Geometry check sheet. Reference: drawing and pictorial views, mm from the part's lowest x, y, z. Round coordinates to 2 decimals unless told otherwise and drop trailing zeros. Write each loop counter-clockwise with the first axis right and the second up, starting at its lowest first coordinate (ties: lowest second). Pieces come first, ordered by that corner, then holes.
Item 1: Section check A-A, the plane z = 17. Record the cut outline in (x, y).
Item 2: Section check B-B, the plane x = 17. Record the cut outline in (y, z).
Item 3: Section check D-D, the plane y = 4.75. Record the cut outline in (x, z), plus the area to 3 significant figures.
Item 4: Section check C-C, the plane y = 0.75. Record the cut outline in (x, z), plus the area to 3 significant figures.
Item 5: Material ranges on line 1 along Z through (x, y) = (17, 2.45); line 2 along Z through (x, y) = (17, 5.3), recorded low to high.
Item 6: Release check for a two-part mould opening along Z. For the marked faces 1, 2 and 3 record: pulls with the +Z half, pulls with the -Z half, needs draft (parallel to the pull), parting line crosses it, or undercut.
Item 7: Depth check by flat-ended pin: pin 1 (10 mm diameter, centred on x = 10, z = 18.5, fed in from +Y); pin 2 (2 mm diameter, centred on x = 30, z = 18.5, fed in from -Y); pin 3 (2 mm diameter, centred on y = 5, z = 9.5, fed in from -X); pin 4 (1.5 mm diameter, centred on y = 5.5, z = 14, fed in from +X). Enter the tip coordinate at first touch or a pass-through.
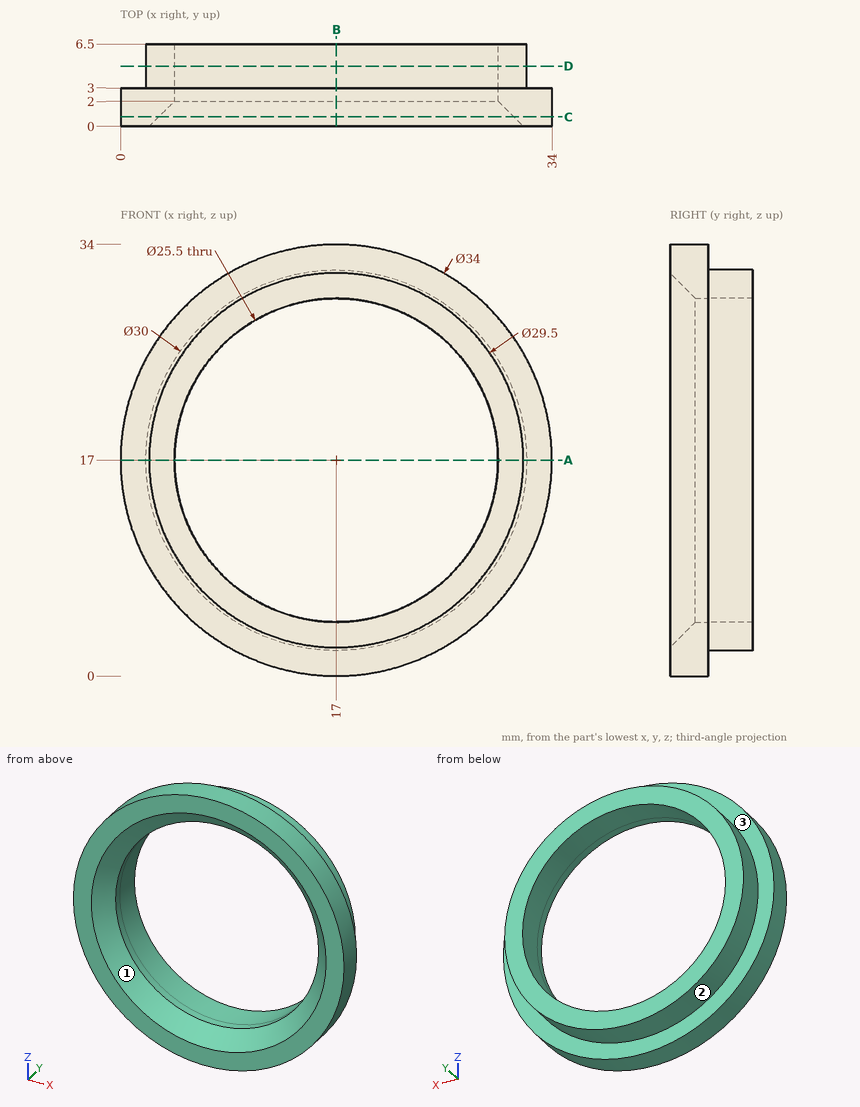
Values found:
1. outline: (0, 0) - (2.25, 0) - (4.25, 2) - (4.25, 6.5) - (2, 6.5) - (2, 3) - (0, 3) - close; (29.75, 2) - (31.75, 0) - (34, 0) - (34, 3) - (32, 3) - (32, 6.5) - (29.75, 6.5) - close
2. outline: (0, 0) - (3, 0) - (3, 2) - (6.5, 2) - (6.5, 4.25) - (2, 4.25) - (0, 2.25) - close; (0, 31.75) - (2, 29.75) - (6.5, 29.75) - (6.5, 32) - (3, 32) - (3, 34) - (0, 34) - close
3. outline: circle Ø30 at (17, 17); hole circle Ø25.5 at (17, 17)
3. area: 196 mm2
4. outline: circle Ø34 at (17, 17); hole circle Ø28 at (17, 17)
4. area: 292 mm2
5. line 1: z = 0 to 4.25, 29.75 to 34
5. line 2: z = 2 to 4.25, 29.75 to 32
6. face 1: undercut
6. face 2: parting line crosses it
6. face 3: needs draft
7. pin 1: passes through
7. pin 2: stops at y = 0.66
7. pin 3: stops at x = 3.48
7. pin 4: stops at x = 31.83
